Part model, mm, in its own coordinate system. Round coordinates to 2 decimals unless told otherwise and drop trailing zeros. One line per question, with ' | ' between items.
from build123d import *

# Parameters (mm, degrees)
SKETCH1_W           = 152.4
SKETCH1_H           = 304.8
BOSS_EXTRUDE1_DEPTH = 1.5748
CUT_EXTRUDE1_REACH  = 172.396
SKETCH2_R           = 2.665


with BuildPart() as part:
    # Sketch1 → Boss-Extrude1 (new body)
    with BuildSketch(Plane.XY):
        Rectangle(SKETCH1_W, SKETCH1_H)
    extrude(amount=BOSS_EXTRUDE1_DEPTH)

    # Sketch2 → Cut-Extrude1 (cut, up to next)
    with BuildSketch(Plane(origin=(0, 0, 0), x_dir=(-1, 0, 0), z_dir=(0, 0, -1)), mode=Mode.PRIVATE) as cut_extrude1_sk1:
        with Locations((-66.2, 137.4)):
            Circle(SKETCH2_R)
    cut_extrude1_tool1 = extrude(cut_extrude1_sk1.sketch, amount=-CUT_EXTRUDE1_REACH, mode=Mode.PRIVATE) & part.part
    # Sketch2 → Cut-Extrude1 (cut, up to next)
    with BuildSketch(Plane(origin=(0, 0, 0), x_dir=(-1, 0, 0), z_dir=(0, 0, -1)), mode=Mode.PRIVATE) as cut_extrude1_sk2:
        with Locations((-66.2, -137.4)):
            Circle(SKETCH2_R)
    cut_extrude1_tool2 = extrude(cut_extrude1_sk2.sketch, amount=-CUT_EXTRUDE1_REACH, mode=Mode.PRIVATE) & part.part
    # Sketch2 → Cut-Extrude1 (cut, up to next)
    with BuildSketch(Plane(origin=(0, 0, 0), x_dir=(-1, 0, 0), z_dir=(0, 0, -1)), mode=Mode.PRIVATE) as cut_extrude1_sk3:
        with Locations((-66.2, 0)):
            Circle(SKETCH2_R)
    cut_extrude1_tool3 = extrude(cut_extrude1_sk3.sketch, amount=-CUT_EXTRUDE1_REACH, mode=Mode.PRIVATE) & part.part
    # Sketch2 → Cut-Extrude1 (cut, up to next)
    with BuildSketch(Plane(origin=(0, 0, 0), x_dir=(-1, 0, 0), z_dir=(0, 0, -1)), mode=Mode.PRIVATE) as cut_extrude1_sk4:
        with Locations((66.2, -137.4)):
            Circle(SKETCH2_R)
    cut_extrude1_tool4 = extrude(cut_extrude1_sk4.sketch, amount=-CUT_EXTRUDE1_REACH, mode=Mode.PRIVATE) & part.part
    # Sketch2 → Cut-Extrude1 (cut, up to next)
    with BuildSketch(Plane(origin=(0, 0, 0), x_dir=(-1, 0, 0), z_dir=(0, 0, -1)), mode=Mode.PRIVATE) as cut_extrude1_sk5:
        with Locations((66.2, 0)):
            Circle(SKETCH2_R)
    cut_extrude1_tool5 = extrude(cut_extrude1_sk5.sketch, amount=-CUT_EXTRUDE1_REACH, mode=Mode.PRIVATE) & part.part
    # Sketch2 → Cut-Extrude1 (cut, up to next)
    with BuildSketch(Plane(origin=(0, 0, 0), x_dir=(-1, 0, 0), z_dir=(0, 0, -1)), mode=Mode.PRIVATE) as cut_extrude1_sk6:
        with Locations((66.2, 137.4)):
            Circle(SKETCH2_R)
    cut_extrude1_tool6 = extrude(cut_extrude1_sk6.sketch, amount=-CUT_EXTRUDE1_REACH, mode=Mode.PRIVATE) & part.part
    add(cut_extrude1_tool1.solids().sort_by_distance((66.2, 137.4, 0))[0], mode=Mode.SUBTRACT)
    add(cut_extrude1_tool2.solids().sort_by_distance((66.2, -137.4, 0))[0], mode=Mode.SUBTRACT)
    add(cut_extrude1_tool3.solids().sort_by_distance((66.2, 0, 0))[0], mode=Mode.SUBTRACT)
    add(cut_extrude1_tool4.solids().sort_by_distance((-66.2, -137.4, 0))[0], mode=Mode.SUBTRACT)
    add(cut_extrude1_tool5.solids().sort_by_distance((-66.2, 0, 0))[0], mode=Mode.SUBTRACT)
    add(cut_extrude1_tool6.solids().sort_by_distance((-66.2, 137.4, 0))[0], mode=Mode.SUBTRACT)


solid = part.part
1) Drop a flat-ended pin along its axis: pin 1 (5 mm diameter, centred on x = -66.2, y = 137.4, fed in from -Z). Give the stop position or say it passes through.
The answers:
pin 1: passes through
2) Probe line 1 (X direction, y = 137.4, z = 0.9) (3 decimals); line 2 (Y direction, x = -66.2, z = 0.4) (3 decimals); line 3 (Y direction, x = -68, z = 1.4). List the from-to ranges inside material, lowest first. Write a range as [from, to].
The answers:
line 1: x = [-76.2, -68.865], [-63.535, 63.535], [68.865, 76.2] | line 2: y = [-152.4, -140.065], [-134.735, -2.665], [2.665, 134.735], [140.065, 152.4] | line 3: y = [-152.4, -139.37], [-135.43, -1.97], [1.97, 135.43], [139.37, 152.4]
3) Two-plate mould, pull along Y, no slides. Class faces 1 (the face through (66.55, -134.76, 0.78)), 2 (the face through (-1, 2, 1.575)): released by +Y, released by -Y, zero draft, split by the parting line, or undercut.
The answers:
face 1: undercut | face 2: zero draft
